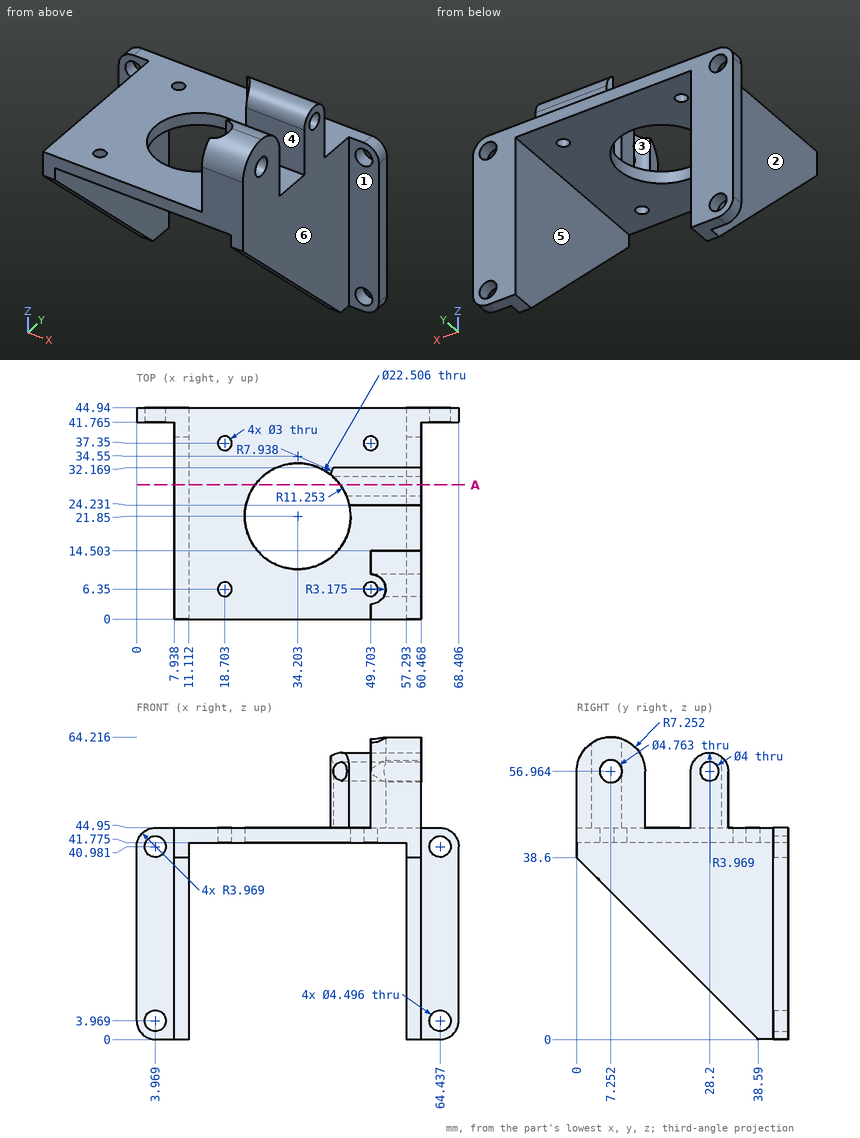
Source: three-view drawing plus pictorial views. Frame: mm from the lowest corner of the part. A direction names the side the tool comes from. Round coordinates to 2 decimals unless told otherwise and drop trailing zeros. Use a Markdown table: item, result.
1. Mould query, pull axis X, two halves, no side actions, for the marked faces 4, 5 and 6. Classes: +X half, -X half, draft (parallel to the pull), parting line (faces both ways), or undercut.
Evaluation:
| item | result |
|---|---|
| face 4 | draft |
| face 5 | undercut |
| face 6 | +X half |
2. Section A-A on y = 28.5. State how many separate pieces and enclosed holes the cut face has, then the cut area to 3 significant figures.
Evaluation:
| item | result |
|---|---|
| separate pieces | 3 |
| enclosed holes | 0 |
| area | 517 mm^2 |
3. First-contact query: pin 1 (5 mm diameter, centred on y = 36.5, z = 21, fed in from -X); pin 2 (3.5 mm diameter, centred on x = 55, z = 52, fed in from +Y); pin 3 (21 mm diameter, centred on y = 14, z = 18, fed in from +X). Flat tips, straight axial feed; report the tip coordinate or a pass-through.
Evaluation:
| item | result |
|---|---|
| pin 1 | x = 7.94 |
| pin 2 | y = 32.17 |
| pin 3 | x = 60.47 |
4. Material intervals for probe 1 along X at (y, z) = (32.5, 36); probe 2 along Y at (x, z) = (46.5, 49); probe 3 along X at (y, z) = (13, 50), sorted ascending.
Evaluation:
| item | result |
|---|---|
| probe 1 | 7.94 to 11.11, 57.29 to 60.47 |
| probe 2 | 24.23 to 32.17 |
| probe 3 | 49.7 to 60.47 |
5. Access query for the marked faces 1, 2 and 3. Directions: +Z, -Z, +X, -X, +Y, -Y. A direction counts if a zero-diameter tool reaches every point of the face in a straight line with its end or side. Return the directions, or none.
Evaluation:
| item | result |
|---|---|
| face 1 | +Z, -Z, +X, -Y |
| face 2 | +Z, -Z, -X, -Y |
| face 3 | +Z, -X |
